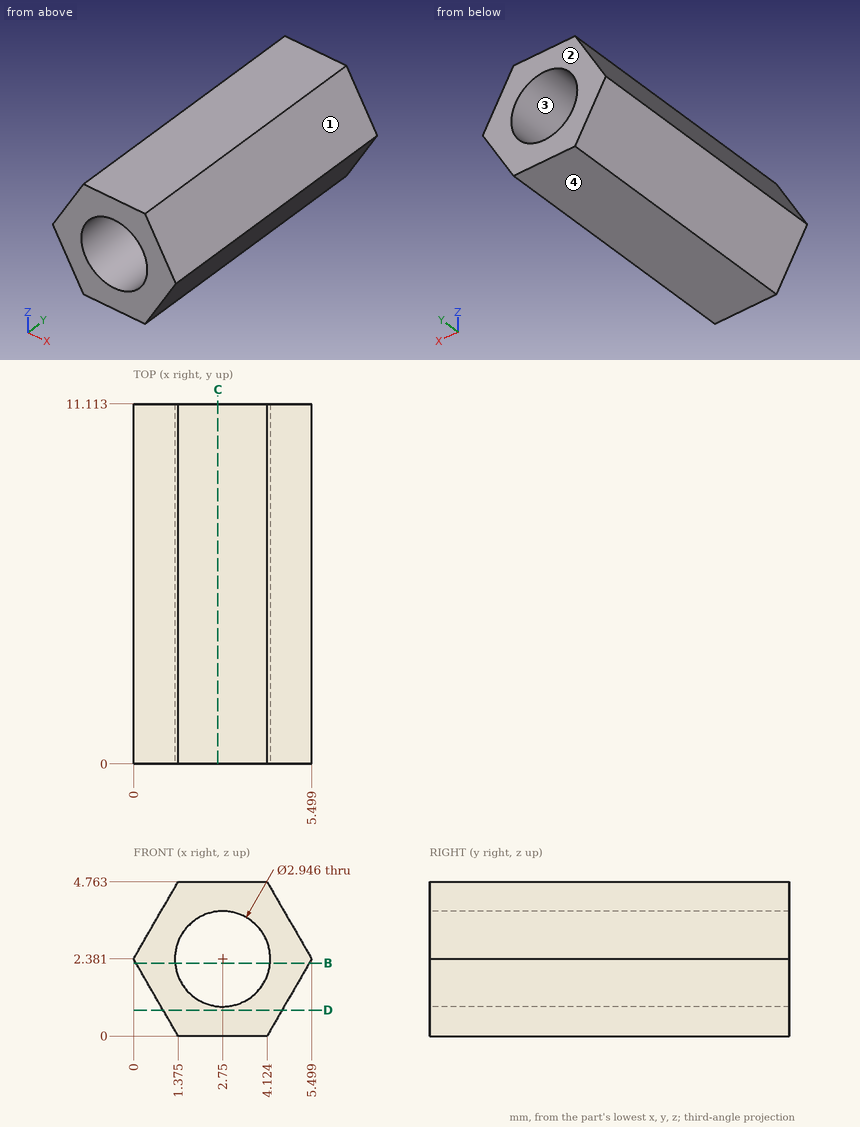
Verification items for this drawing (mm, ordinates from the low corner). Give positions to 0.01 mm unless a question says otherwise; leave off trailing zeros. Write each loop counter-clockwise with the first axis right and the second up, starting at its lowest first coordinate (ties: lowest second). Pieces come first, ordered by that corner, then holes.
1) Release check for a two-part mould opening along Z. For the marked faces 1, 2, 3 and 4 record: pulls with the +Z half, pulls with the -Z half, needs draft (parallel to the pull), parting line crosses it, or undercut.
2) Section check C-C, the plane x = 2.6. Record the boundary of the cut face in (y, z) (1 decimal).
3) Section check D-D, the plane z = 0.8. Record the boundary of the cut face in (x, y).
4) Section check B-B, the plane z = 2.25. Record the boundary of the cut face in (x, y) (1 decimal).
5) Material ranges on L1, parallel to Z at x = 2.7, y = 1.75; L2, parallel to X at y = 2.5, z = 1.7 (1 decimal); L3, parallel to X at y = 5, z = 2.65 (1 decimal), recorded low to high.
Computed:
1. face 1: pulls with the +Z half
1. face 2: needs draft
1. face 3: undercut
1. face 4: pulls with the -Z half
2. outline: (0, 0) - (11.1, 0) - (11.1, 0.9) - (0, 0.9) - close; (0, 3.8) - (11.1, 3.8) - (11.1, 4.8) - (0, 4.8) - close
3. outline: (0.91, 0) - (4.59, 0) - (4.59, 11.11) - (0.91, 11.11) - close
4. outline: (0.1, 0) - (1.3, 0) - (1.3, 11.1) - (0.1, 11.1) - close; (4.2, 0) - (5.4, 0) - (5.4, 11.1) - (4.2, 11.1) - close
5. L1: z = 0 to 0.91, 3.85 to 4.76
5. L2: x = 0.4 to 1.4, 4.1 to 5.1
5. L3: x = 0.2 to 1.3, 4.2 to 5.3
